Verification items for the finished model (mm, model axes). A direction names the side the tool comes from. Give positions to 0.01 mm unless a question says otherwise; leave off trailing zeros. Write each loop counter-clockwise with the first axis right and the second up, starting at its lowest first coordinate (ties: lowest second). Pieces come first, ordered by that corner, then holes. Notation, with made-up numbers: (68, 71.5) -> (76, 71.5) arc R22 cw to (76, 98.5) -> close; hole circle Ø9 at (-23.75, 18.5). An arc over 180 degrees is marked (long way). Answer as CSV lines item,"result". Start each with the question number.
1) Tool access check on faces 1 (the flat face through (-0.661, 1.726, -2.926)), 2 (the flat face through (-2.75, 5, -9)), 3 (the flat face through (2.865, 1.726, 0.891)), 4 (the flat face through (0, 6, 2.1)), 5 (the flat face through (-2, 4, -6)). Record the directions out of +Z, -Z, +X, -X, +Y, -Y that give a thin tool (end or side, any length) a straight path to the whole face; none if there is none.
2) Sectioned sample at D-D on y = 6.25. Record the cut outline in (x, z).
3) Sectioned sample at C-C on x = 0. Record the cut outline in (y, z), and give its area (3 significant figures).
4) Sectioned sample at A-A on z = 0.25. Record the cut outline in (x, y), and give its area (3 significant figures).
5) Material ranges on L1, parallel to Y at x = -6.5, z = -4.5; L2, parallel to X at y = 2.25, z = 0; L3, parallel to X at y = 1.5, z = -1.25, recorded low to high.
6) Sectioned sample at B-B on y = 1. Record the cut outline in (x, z).
7) Mould release check, pull along X, two halves, no side actions. Record for faces 6 (the cylindrical face through (0, 5, 10)), 7 (the flat face through (2.75, 5, -9)), 8 (the flat face through (0.661, 1.726, 2.926)), 9 (the cylindrical face through (-3.1, 6, 0)): released by +X, released by -X, zero draft, split by the parting line, or undercut.
8) Gauge pin test, flat ends, axial feed: pin 1 Ø1.5 at (x, y) = (0.5, 5.5) entering from -Z; pin 2 Ø2 at (y, z) = (2, 0.5) entering from +X; pin 3 Ø1.3 at (x, z) = (0, 0.5) entering from +Y; pin 4 Ø4 at (y, z) = (3, 4) entering from -X. Record the tip position at first contact, or that the pin passes through.
```python
from build123d import *

# Parameters (mm, degrees)
EXTRUDE_1_DEPTH     = 3.5
EXTRUDE_2_DEPTH     = 4
SKETCH_4_R          = 1.5
CUT_EXTRUDE_1_DEPTH = 4
CUT_EXTRUDE_2_DEPTH = 3
SKETCH_6_R          = 1.5
CUT_EXTRUDE_3_DEPTH = 17.007810594
SKETCH_7_W          = 4
SKETCH_7_H          = 4.5
CUT_EXTRUDE_4_DEPTH = 0.9
SKETCH_8_W          = 4
SKETCH_8_H          = 4.5
EXTRUDE_3_DEPTH     = 0.9


with BuildPart() as part:
    # 草图1 → 凸台-拉伸1 (new body)
    with BuildSketch(Plane(origin=(0, 0, 0), x_dir=(1, 0, 0), z_dir=(0, 1, 0))):
        Polygon((2.370649369, -2.525870458), (3.372792668, 0.790107348), (1.002143299, 3.315977806), (-2.370649369, 2.525870458), (-3.372792668, -0.790107348), (-1.002143299, -3.315977806), align=None)
    extrude(amount=EXTRUDE_1_DEPTH)

    # 草图3 → 凸台-拉伸2 (add)
    with BuildSketch(Plane(origin=(0, 3.5, 0), x_dir=(1, 0, 0), z_dir=(0, 1, 0))):
        with BuildLine():
            Line((-2.75, 8), (2.75, 8))
            Line((2.75, 8), (2.75, 9.614442262))
            ThreePointArc((2.75, 9.614442262), (0, -10), (-2.75, 9.614442262))
            Line((-2.75, 9.614442262), (-2.75, 8))
        make_face()
    extrude(amount=EXTRUDE_2_DEPTH)

    # 草图4 → 切除-拉伸1 (cut)
    with BuildSketch(Plane.XZ):
        with Locations(Location((0, 0, 0), (0, 0, 270))):
            Circle(SKETCH_4_R)
    extrude(amount=-CUT_EXTRUDE_1_DEPTH, mode=Mode.SUBTRACT)

    # 草图5 → 切除-拉伸2 (cut)
    with BuildSketch(Plane(origin=(0, 7.5, 0), x_dir=(1, 0, 0), z_dir=(0, 1, 0))):
        with BuildLine():
            Line((-2.28035085, 2.1), (2.28035085, 2.1))
            ThreePointArc((2.28035085, 2.1), (3.1, 0), (2.28035085, -2.1))
            Line((2.28035085, -2.1), (-2.28035085, -2.1))
            ThreePointArc((-2.28035085, -2.1), (-3.1, 0), (-2.28035085, 2.1))
        make_face()
    extrude(amount=-CUT_EXTRUDE_2_DEPTH, mode=Mode.SUBTRACT)

    # 草图6 → 切除-拉伸3 (cut, through all)
    with BuildSketch(Plane.XZ):
        with Locations(Location((0, 0, 0), (0, 0, 270))):
            Circle(SKETCH_6_R)
    extrude(amount=-CUT_EXTRUDE_3_DEPTH, mode=Mode.SUBTRACT)

    # 草图7 → 切除-拉伸4 (cut)
    with BuildSketch(Plane(origin=(0, 7.5, 0), x_dir=(1, 0, 0), z_dir=(0, 1, 0))):
        with Locations((0, 5.75)):
            Rectangle(SKETCH_7_W, SKETCH_7_H)
    cut_extrude_4 = extrude(amount=-CUT_EXTRUDE_4_DEPTH, mode=Mode.SUBTRACT)

    # 镜向1: 切除-拉伸4 across plane
    add(cut_extrude_4.mirror(Plane.ZX.offset(5.5)), mode=Mode.SUBTRACT)

    # 草图8 → 凸台-拉伸3 (add)
    with BuildSketch(Plane(origin=(0, 6.6, 0), x_dir=(1, 0, 0), z_dir=(0, 1, 0))):
        with Locations((0, 5.75)):
            Rectangle(SKETCH_8_W, SKETCH_8_H)
    extrude(amount=EXTRUDE_3_DEPTH)


solid = part.part
```
Ans:
1,face 1,"-Z, -X, -Y"
1,face 2,"-Z, +Y, -Y"
1,face 3,"+Z, +X, -Y"
1,face 4,"+Y"
1,face 5,"-Z, -Y"
2,outline,"(-2.75, -9.61) -> (-2.75, -8) -> (2.75, -8) -> (2.75, -9.61) arc R10 ccw (long way) to start; hole (-2.28, -2.1) -> (2.28, -2.1) arc R3.1 ccw to (2.28, 2.1) -> (-2.28, 2.1) arc R3.1 ccw to start"
3,outline,"(0, -3.08) -> (3.5, -3.08) -> (3.5, -3.5) -> (4.4, -3.5) -> (4.4, -8) -> (7.5, -8) -> (7.5, -2.1) -> (4.5, -2.1) -> (4.5, -1.5) -> (0, -1.5) -> close; (0, 1.5) -> (4.5, 1.5) -> (4.5, 2.1) -> (7.5, 2.1) -> (7.5, 10) -> (3.5, 10) -> (3.5, 3.08) -> (0, 3.08) -> close"
3,area,"63.4 mm²"
4,outline,"(-10, 3.5) -> (-3.21, 3.5) -> (-3.21, 0) -> (-1.48, 0) -> (-1.48, 4.5) -> (-3.09, 4.5) -> (-3.09, 7.5) -> (-10, 7.5) -> close; (1.48, 0) -> (3.06, 0) -> (3.06, 3.5) -> (10, 3.5) -> (10, 7.5) -> (3.09, 7.5) -> (3.09, 4.5) -> (1.48, 4.5) -> close"
4,area,"70.1 mm²"
5,L1,"y = 3.5 to 7.5"
5,L2,"x = -3.13 to -1.5, 1.5 to 3.13"
5,L3,"x = -2.76 to -0.83, 0.83 to 2.94"
6,outline,"(-3.37, 0.79) -> (-2.37, -2.53) -> (1, -3.32) -> (3.37, -0.79) -> (2.37, 2.53) -> (-1, 3.32) -> close; hole circle Ø3 at (0, 0)"
7,face 6,"split by the parting line"
7,face 7,"undercut"
7,face 8,"released by +X"
7,face 9,"undercut"
8,pin 1,"stops at z = -8"
8,pin 2,"stops at x = 3.29"
8,pin 3,"passes through"
8,pin 4,"stops at x = -9.78"
